```python
from build123d import *

# Parameters (mm, degrees)
SKETCH1_R                   = 2.05
SKETCH1_R_2                 = 1.5
BOSS_EXTRUDE1_DEPTH         = 5.5
FILLET1_START               = -1
FILLET1_DEPTH               = 7
FILLET1_2_DEPTH             = 5.5
TAP_DRILL_FOR_M2X0_4_TAP1_D = 1.6
SKETCH4_W                   = 9
SKETCH4_H                   = 9
CUT_EXTRUDE1_DEPTH          = 2
SKETCH5_R                   = 5
CUT_EXTRUDE2_DEPTH          = 3.5


with BuildPart() as part:
    # Sketch1 → Boss-Extrude1 (new body)
    with BuildSketch(Plane(origin=(0, 0, 0), x_dir=(0, 0, -1), z_dir=(1, 0, 0))):
        with BuildLine():
            Line((6, 0), (6, 28))
            ThreePointArc((6, 28), (4.242640687, 32.242640687), (0, 34))
            Line((0, 34), (-9.875644347, 34))
            ThreePointArc((-9.875644347, 34), (-14.875644347, 35.339745962), (-18.535898385, 39))
            Line((-18.535898385, 39), (-21.084936491, 43.415063509))
            Line((-21.084936491, 43.415063509), (-25.415063509, 40.915063509))
            Line((-25.415063509, 40.915063509), (-17.260063509, 26.790189174))
            ThreePointArc((-17.260063509, 26.790189174), (-16.528012702, 26.058138366), (-15.528012702, 25.790189174))
            Line((-15.528012702, 25.790189174), (-13, 25.790189174))
            ThreePointArc((-13, 25.790189174), (-5.928932188, 22.861256986), (-3, 15.790189174))
            Line((-3, 15.790189174), (-3, 3))
            Line((-3, 3), (-5, 3))
            Line((-5, 3), (-5, -3.31662479))
            ThreePointArc((-5, -3.31662479), (1.732050808, -5.744562647), (6, 0))
        make_face()
        Circle(SKETCH1_R, mode=Mode.SUBTRACT)
        with Locations((-22, 40)):
            Circle(SKETCH1_R_2, mode=Mode.SUBTRACT)
        with Locations((-17, 31.339745962)):
            Circle(SKETCH1_R_2, mode=Mode.SUBTRACT)
        with Locations((-1, 11.5)):
            Circle(SKETCH1_R_2, mode=Mode.SUBTRACT)
        with Locations((4, 11.5)):
            Circle(SKETCH1_R_2, mode=Mode.SUBTRACT)
        with Locations((4, 7.5)):
            Circle(SKETCH1_R_2, mode=Mode.SUBTRACT)
    extrude(amount=BOSS_EXTRUDE1_DEPTH)

    # Fillet1: read off the stored shape, not the designer's step
    # Fillet1 outline → Fillet1 (cut)
    with BuildSketch(Plane.YZ.offset(FILLET1_START)):
        with BuildLine():
            ThreePointArc((2, 5), (2.707106781, 4.707106781), (3, 4))
            Line((3, 4), (3, 5))
            Line((3, 5), (2, 5))
        make_face()
    extrude(amount=FILLET1_DEPTH, mode=Mode.SUBTRACT)

    # Fillet1 2 outline → Fillet1 2 (add)
    with BuildSketch(Plane.YZ):
        with BuildLine():
            ThreePointArc((4, 3), (3.292893219, 3.292893219), (3, 4))
            Line((3, 4), (3, 3))
            Line((3, 3), (4, 3))
        make_face()
    extrude(amount=FILLET1_2_DEPTH)

    # Tap Drill for M2x0.4 Tap1 (through all)
    with Locations(Plane(origin=(5.5, 0, 0), x_dir=(0, 0, -1), z_dir=(1, 0, 0))):
        with Locations((-1.2, 17), (4, 17)):
            Hole(TAP_DRILL_FOR_M2X0_4_TAP1_D / 2)

    # Sketch4 → Cut-Extrude1 (cut)
    with BuildSketch(Plane.ZY):
        with Locations((-1.5, 9.5)):
            Rectangle(SKETCH4_W, SKETCH4_H)
    extrude(amount=-CUT_EXTRUDE1_DEPTH, mode=Mode.SUBTRACT)

    # Sketch5 → Cut-Extrude2 (cut)
    with BuildSketch(Plane(origin=(5.5, 0, 0), x_dir=(0, 0, -1), z_dir=(1, 0, 0))):
        with Locations((0, 28)):
            Circle(SKETCH5_R)
    extrude(amount=-CUT_EXTRUDE2_DEPTH, mode=Mode.SUBTRACT)


solid = part.part
```
Build history of the part. All positions in model axes, mm. A direction names the side the tool comes from. Round coordinates to 2 decimals unless told otherwise and drop trailing zeros. Write each loop counter-clockwise with the first axis right and the second up, starting at its lowest first coordinate (ties: lowest second). Pieces come first, ordered by that corner, then holes. Notation, with made-up numbers: (-6.75, -32) -> (48.25, -32) arc R32 cw to (48.25, 5) -> close; hole circle Ø9 at (69, -21.75). An arc over 180 degrees is marked (long way). Put each result on its own line as item: value.
Item 1: Slice it at A-A, the plane y = 11.5. Give the cut face in (x, z).
Here are the results:
outline: (2, -6) -> (5.5, -6) -> (5.5, -5.5) -> (2, -5.5) -> close; (2, -2.5) -> (5.5, -2.5) -> (5.5, -0.5) -> (2, -0.5) -> close; (2, 2.5) -> (5.5, 2.5) -> (5.5, 3) -> (2, 3) -> close
Item 2: Two-plate mould, pull along Z, no slides. Class faces 1 (the face through (3.73, 6.17, -4.69)), 2 (the face through (2.71, 22.94, 6.01)), 3 (the face through (2.71, 16.22, -4.17)), 4 (the face through (2.712, 32.196, -4.289)): pulls with the +Z half, pulls with the -Z half, needs draft (parallel to the pull), parting line crosses it, or undercut.
Here are the results:
face 1: undercut
face 2: pulls with the +Z half
face 3: undercut
face 4: pulls with the -Z half
Item 3: Slice it at D-D, the plane y = 6.5. Give the cut face in (x, z), plus the area to 3 significant figures.
Here are the results:
outline: (2, -6) -> (5.5, -6) -> (5.5, -5.12) -> (2, -5.12) -> close; (2, -2.88) -> (5.5, -2.88) -> (5.5, 3) -> (2, 3) -> close
area: 23.7 mm^2
Item 4: Slice it at B-B, the plane x = 0.8. Give the cut face in (y, z).
Here are the results:
outline: (-3.32, 5) arc R6 ccw to (0, -6) -> (5, -6) -> (5, 3) -> (4, 3) arc R1 cw to (3, 4) arc R1 ccw to (2, 5) -> close; (14, -6) -> (28, -6) arc R6 ccw to (34, 0) -> (34, 9.88) arc R10 cw to (39, 18.54) -> (43.42, 21.08) -> (40.92, 25.42) -> (26.79, 17.26) arc R2 ccw to (25.79, 15.53) -> (25.79, 13) arc R10 cw to (15.79, 3) -> (14, 3) -> close; hole circle Ø4.1 at (0, 0); hole circle Ø1.6 at (17, -4); hole circle Ø1.6 at (17, 1.2); hole circle Ø3 at (31.34, 17); hole circle Ø3 at (40, 22)
Item 5: Flat gauge pins, fed straight in: P1, Ø3, axis at x = 2, z = 0.5, coming from the +Y side; P2, Ø8, axis at y = 28, z = 0, coming from the +X side; P3, Ø1.5, axis at x = 1.5, z = 12, coming from the -Y side; P4, Ø5, axis at y = 10.5, z = 2, coming from the +X side. Where does each tip first touch, or does it go through?
Here are the results:
P1: stops at y = 34
P2: stops at x = 2
P3: stops at y = 25.64
P4: stops at x = 5.5
Item 6: Wall check: probe 1 along Y at (x, z) = (3.35, 1); probe 2 along Y at (x, z) = (3, 1.2); probe 3 along Y at (x, z) = (2.85, 0). Give the ranges that are in metal, low to high. Write a range as from..to.
Here are the results:
probe 1: y = -5.92..-1.79, 1.79..10, 13..16.23, 17.77..23.1, 32.9..34
probe 2: y = -5.88..-1.66, 1.66..10.01, 12.99..16.2, 17.8..23.15, 32.85..34
probe 3: y = -6..-2.05, 2.05..10.38, 12.62..23, 33..34
Item 7: Tool access for faces 5 (the face through (3.77, 23.12, 1.08)), 6 (the face through (3, 25.79, 14)), 7 (the face through (1, 14, -2)): list every direction of +Z, -Z, +X, -X, +Y, -Y with a clear straight run to the whole face (end or side of a thin tool).
Here are the results:
face 5: +X
face 6: +Z, +X, -X, -Y
face 7: +Z, -Z, -X
Item 8: Slice it at C-C, the plane z = 16.5. Give the cut face in (x, y).
Here are the results:
outline: (0, 26.04) -> (5.5, 26.04) -> (5.5, 29.93) -> (0, 29.93) -> close; (0, 32.75) -> (5.5, 32.75) -> (5.5, 36.51) -> (0, 36.51) -> close
